Geometry check sheet. Reference: drawing and pictorial views, mm from the part's lowest x, y, z. A direction names the side the tool comes from. Coordinates: 2 decimals unless noted, no trailing zeros. Loops run counter-clockwise (first coordinate to the right, second up) from the corner with the lowest first, then second, coordinate; pieces in that order, holes last. Notation, with made-up numbers: (88, 28.5) -> (96, 28.5) arc R18 ccw to (96, 60.5) -> close; hole circle Ø8 at (-26.5, -35.75). An arc over 180 degrees is marked (long way). Answer as a JSON object with one key per item and string values. Group by question number.
Q1. Cross-section at B-B on z = 11. Record the boundary of the cut face in (x, y).
Q2. Scan lines: L1, parallel to Z at x = 63.5, y = 15.75; L2, parallel to X at y = 9, z = 72.5 (1 decimal); L3, parallel to Y at x = 74, z = 68 (1 decimal). Record each from-to range of solid material in increasing order.
Q3. Cross-section at A-A on x = 63.5. Give the number of separate pieces and of enclosed holes in the cut face, and give its area (3 significant figures).
Q4. Set-up check for the marked faces 4 and 5: record each of +Z, -Z, +X, -X, +Y, -Y from which the full face is reachable in a straight line by a thin tool's end or side.
Q5. Release check for a two-part mould opening along X. For the marked faces 1, 2 and 3 record: released by +X, released by -X, zero draft, split by the parting line, or undercut.
Q6. Gauge pin test, flat ends, axial feed: pin 1 Ø3 at (x, z) = (82, 19) entering from +Y; pin 2 Ø12 at (y, z) = (16, 12) entering from +X; pin 3 Ø12 at (x, z) = (40, 65.5) entering from -Y; pin 4 Ø14 at (x, z) = (63.5, 15.1) entering from +Y. Record the tip position at first contact, or that the pin passes through.
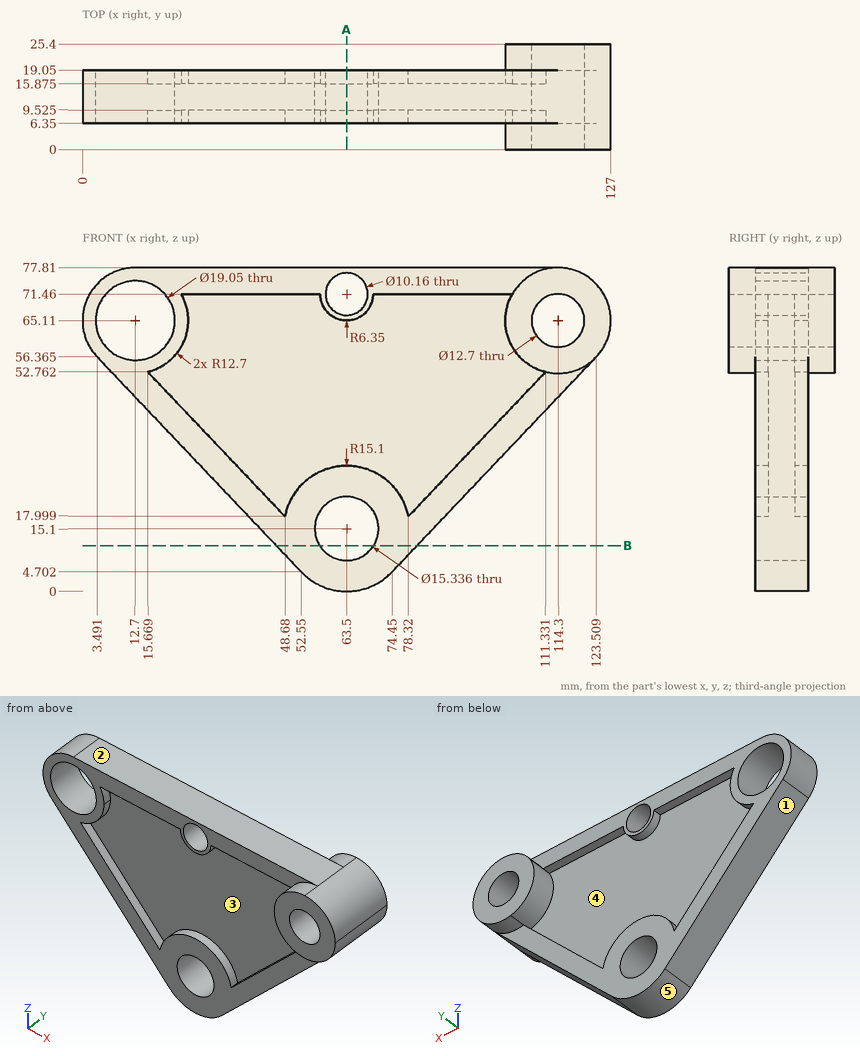
Computed values:
{
 "1": {"outline": "(46.57, 6.35) -> (57.02, 6.35) -> (57.02, 19.05) -> (46.57, 19.05) -> close; (69.98, 6.35) -> (80.43, 6.35) -> (80.43, 19.05) -> (69.98, 19.05) -> close"},
 "2": {"L1": "z = 0 to 7.43, 22.77 to 66.38, 76.54 to 77.81", "L2": "x = 2.4 to 6.7, 18.7 to 58.5, 68.5 to 124.6", "L3": "y = 9.5 to 15.9"},
 "3": {"separate pieces": "3", "enclosed holes": "0", "area": "443 mm²"},
 "4": {"face 4": "+Y", "face 5": "-Z, +Y, -Y"},
 "5": {"face 1": "released by -X", "face 2": "zero draft", "face 3": "undercut"},
 "6": {"pin 1": "stops at y = 19.05", "pin 2": "stops at x = 87.08", "pin 3": "stops at y = 6.35", "pin 4": "passes through"}
}
